from build123d import *

# Parameters (mm, degrees)
SKETCH1_W                         = 150
SKETCH1_H                         = 50
BOSS_EXTRUDE1_DEPTH               = 10
SKETCH2_R                         = 1.5
LINEAR_BEARING_MOUNT_DEPTH        = 11
SKETCH3_R                         = 2.5
SURFACE_PROFILE_MOUNT_DEPTH       = 11
SKETCH4_R                         = 4.25
SURF_PROF_MOUNT_COUNTERSINK_DEPTH = 5
SKETCH5_R                         = 3.5
CUT_EXTRUDE1_DEPTH                = 4


with BuildPart() as part:
    # Sketch1 → Boss-Extrude1 (new body)
    with BuildSketch(Plane(origin=(0, 0, 0), x_dir=(1, 0, 0), z_dir=(0, 1, 0))):
        Rectangle(SKETCH1_W, SKETCH1_H)
    extrude(amount=BOSS_EXTRUDE1_DEPTH)

    # Sketch2 → Linear_bearing_mount (cut, through all)
    with BuildSketch(Plane(origin=(0, 10, 0), x_dir=(1, 0, 0), z_dir=(0, 1, 0))):
        with Locations((-43, -12)):
            Circle(SKETCH2_R)
        with Locations((-61, -12)):
            Circle(SKETCH2_R)
        with Locations((43, -12)):
            Circle(SKETCH2_R)
        with Locations((61, -12)):
            Circle(SKETCH2_R)
        with Locations((61, 12)):
            Circle(SKETCH2_R)
        with Locations((43, 12)):
            Circle(SKETCH2_R)
        with Locations((-61, 12)):
            Circle(SKETCH2_R)
        with Locations((-43, 12)):
            Circle(SKETCH2_R)
    extrude(amount=-LINEAR_BEARING_MOUNT_DEPTH, mode=Mode.SUBTRACT)

    # Sketch3 → Surface_profile_mount (cut, through all)
    with BuildSketch(Plane.XZ):
        Circle(SKETCH3_R)
        with Locations((45, 0)):
            Circle(SKETCH3_R)
        with Locations((-30, 0)):
            Circle(SKETCH3_R)
    extrude(amount=-SURFACE_PROFILE_MOUNT_DEPTH, mode=Mode.SUBTRACT)

    # Sketch4 → Surf.prof.mount_countersink (cut)
    with BuildSketch(Plane.XZ):
        with Locations((45, 0)):
            Circle(SKETCH4_R)
        Circle(SKETCH4_R)
        with Locations((-30, 0)):
            Circle(SKETCH4_R)
    extrude(amount=-SURF_PROF_MOUNT_COUNTERSINK_DEPTH, mode=Mode.SUBTRACT)

    # Sketch5 → Cut-Extrude1 (cut)
    with BuildSketch(Plane(origin=(0, 10, 0), x_dir=(1, 0, 0), z_dir=(0, 1, 0))):
        with Locations((-61, 12)):
            Circle(SKETCH5_R)
        with Locations((-43, 12)):
            Circle(SKETCH5_R)
        with Locations((-43, -12)):
            Circle(SKETCH5_R)
        with Locations((-61, -12)):
            Circle(SKETCH5_R)
        with Locations((61, -12)):
            Circle(SKETCH5_R)
        with Locations((43, -12)):
            Circle(SKETCH5_R)
        with Locations((43, 12)):
            Circle(SKETCH5_R)
        with Locations((61, 12)):
            Circle(SKETCH5_R)
    extrude(amount=-CUT_EXTRUDE1_DEPTH, mode=Mode.SUBTRACT)


solid = part.part
Geometry: final body of the model. Coordinates: model frame, mm. A direction names the side the tool comes from. Round coordinates to 2 decimals unless told otherwise and drop trailing zeros. Loops run counter-clockwise (first coordinate to the right, second up) from the corner with the lowest first, then second, coordinate; pieces in that order, holes last. Notation, with made-up numbers: M -24,69.5 L 33,69.5 A25 ccw 33,90.5 Z; hole C 25.25,85 d2. An arc over 180 degrees is marked long. Put each result on its own line as item: value. Start each with the question number.
(1) Section query A-A (x = 0). Return loops of the section in (y, z).
(2) Contact query for flat-ended pins moving along their axis: pin 1 Ø3.5 at (x, z) = (-61, -12.5) entering from +Y; pin 2 Ø1.8 at (x, z) = (-61, 12) entering from +Y; pin 3 Ø6.5 at (x, z) = (45, 0) entering from -Y. Output: stop coordinate, or through.
(3) Section query C-C (z = 0). Return loops of the section in (x, y).
(4) Set-up query: faces 1 (the face through (2.285, 2.465, 3.584)), 2 (the face through (-59, 6, 12)), 3 (the face through (-59.57, 3.04, -12.45)). Return all of +Z, -Z, +X, -X, +Y, -Y with unobstructed straight access to the full face (end or side cutting, diameter ignored); none if empty.
(5) Section query D-D (z = -12). State how many separate pieces and enclosed holes the cut face has, then the cut area to 3 significant figures.
(6) Draft query along X for faces 4 (the face through (75, 5, 0)), 5 (the face through (-75, 5, 0)), 6 (the face through (40.2, 8, 14.1)). Return one class per face: +X half, -X half, draft (parallel to the pull), parting line (faces both ways), or undercut.
(7) Material intervals for line 1 along Z through (x, y) = (61, 2.05); line 2 along X through (y, z) = (6.5, 12); line 3 along X through (y, z) = (4.3, -12), sorted ascending. Write a range as [from, to].
(8) Section query B-B (x = -61). Return loops of the section in (y, z), then the cut area to 3 significant figures.
Findings below:
1. outline: M 0,-25 L 10,-25 L 10,-2.5 L 5,-2.5 L 5,-4.25 L 0,-4.25 Z; M 0,4.25 L 5,4.25 L 5,2.5 L 10,2.5 L 10,25 L 0,25 Z
2. pin 1: stops at y = 6
2. pin 2: passes through
2. pin 3: stops at y = 5
3. outline: M -75,0 L -34.25,0 L -34.25,5 L -32.5,5 L -32.5,10 L -75,10 Z; M -27.5,5 L -25.75,5 L -25.75,0 L -4.25,0 L -4.25,5 L -2.5,5 L -2.5,10 L -27.5,10 Z; M 2.5,5 L 4.25,5 L 4.25,0 L 40.75,0 L 40.75,5 L 42.5,5 L 42.5,10 L 2.5,10 Z; M 47.5,5 L 49.25,5 L 49.25,0 L 75,0 L 75,10 L 47.5,10 Z
4. face 1: -Y
4. face 2: +Y
4. face 3: +Y, -Y
5. separate pieces: 5
5. enclosed holes: 0
5. area: 1,320 mm2
6. face 4: +X half
6. face 5: -X half
6. face 6: undercut
7. line 1: z = [-25, -13.5], [-10.5, 10.5], [13.5, 25]
7. line 2: x = [-75, -64.5], [-57.5, -46.5], [-39.5, 39.5], [46.5, 57.5], [64.5, 75]
7. line 3: x = [-75, -62.5], [-59.5, -44.5], [-41.5, 41.5], [44.5, 59.5], [62.5, 75]
8. outline: M 0,-25 L 10,-25 L 10,-15.5 L 6,-15.5 L 6,-13.5 L 0,-13.5 Z; M 0,-10.5 L 6,-10.5 L 6,-8.5 L 10,-8.5 L 10,8.5 L 6,8.5 L 6,10.5 L 0,10.5 Z; M 0,13.5 L 6,13.5 L 6,15.5 L 10,15.5 L 10,25 L 0,25 Z
8. area: 408 mm2
